Check sheet for the drawn part. Datum: minimum x, y, z corner. Units: mm. A direction names the side the tool comes from. Round coordinates to 2 decimals unless told otherwise and drop trailing zeros. Write each loop counter-clockwise with the first axis right and the second up, starting at its lowest first coordinate (ties: lowest second). Pieces come first, ordered by that corner, then holes. Notation, with made-up numbers: M -14.75,-20 L 25.25,-20 A23 cw 25.25,-3 Z; hole C 88.5,4.25 d10. An arc over 180 degrees is marked long. Put each result on its own line as item: value.
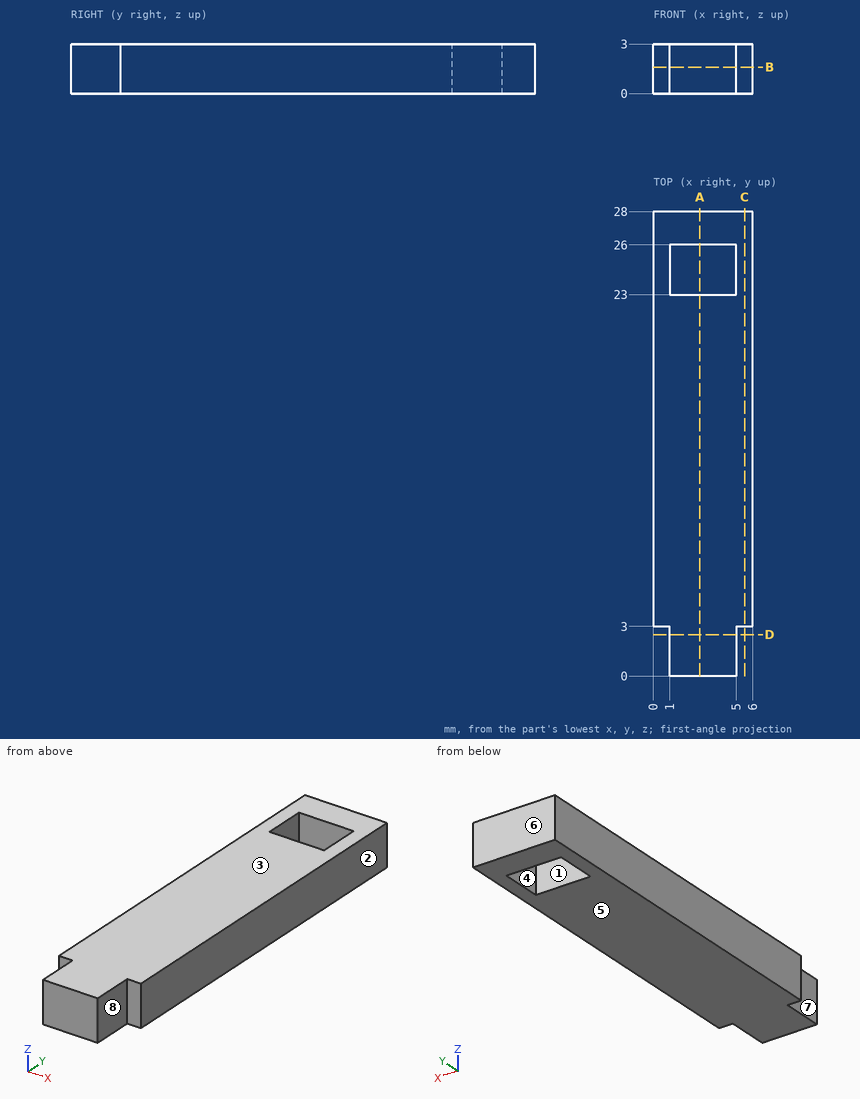
1. Release check for a two-part mould opening along X. For the marked faces 1, 2 and 3 record: +X half, -X half, draft (parallel to the pull), parting line (faces both ways), or undercut.
Computed values:
face 1: undercut
face 2: +X half
face 3: draft
2. Cross-section at C-C (x = 5.5). Enter the section's corners in (y, z), then the cut area to 3 significant figures.
Computed values:
outline: M 3,0 L 28,0 L 28,3 L 3,3 Z
area: 75.0 mm2
3. Access from +Z, -Z, +X, -X, +Y, -Y to the whole of each face (thin tool, end or side, straight path). Record for the marked faces 4, 5, 6, 7 and 8.
Computed values:
face 4: +Z, -Z
face 5: -Z, +X, -X, +Y, -Y
face 6: +Z, -Z, +X, -X, +Y
face 7: +Z, -Z, -X, -Y
face 8: +Z, -Z, +X, -Y
4. Cross-section at A-A (x = 2.8). Enter the section's corners in (y, z), then the cut area to 3 significant figures.
Computed values:
outline: M 0,0 L 23,0 L 23,3 L 0,3 Z; M 26,0 L 28,0 L 28,3 L 26,3 Z
area: 75.0 mm2
5. Depth check by flat-ended pin: pin 1 Ø0.9 at (y, z) = (1.5, 1) entering from -X; pin 2 Ø0.5 at (x, z) = (0.5, 1.5) entering from -Y; pin 3 Ø0.9 at (y, z) = (1, 1.5) entering from +X. Enter the tip coordinate at first touch or a pass-through.
Computed values:
pin 1: stops at x = 1
pin 2: stops at y = 3
pin 3: stops at x = 5
6. Scan lines: probe 1 along Y at (x, z) = (4.8, 0.85); probe 2 along X at (y, z) = (25.25, 1.95); probe 3 along Y at (x, z) = (5.25, 0.85). Record each from-to range of solid material in increasing order.
Computed values:
probe 1: y = 0 to 23, 26 to 28
probe 2: x = 0 to 1, 5 to 6
probe 3: y = 3 to 28
7. Cross-section at B-B (z = 1.6). Enter the section's corners in (x, y), then the cut area to 3 significant figures.
Computed values:
outline: M 0,3 L 1,3 L 1,0 L 5,0 L 5,3 L 6,3 L 6,28 L 0,28 Z; hole M 1,23 L 5,23 L 5,26 L 1,26 Z
area: 150 mm2
8. Cross-section at D-D (y = 2.5). Enter the section's corners in (x, z), then the cut area to 3 significant figures.
Computed values:
outline: M 1,0 L 5,0 L 5,3 L 1,3 Z
area: 12.0 mm2
